Verification items for the finished model (mm, model axes). A direction names the side the tool comes from. Give positions to 0.01 mm unless a question says otherwise; leave off trailing zeros. Loops run counter-clockwise (first coordinate to the right, second up) from the corner with the lowest first, then second, coordinate; pieces in that order, holes last. Notation, with made-up numbers: (25.25, 31.5) - (61.25, 31.5) arc R33 cw to (61.25, 64.5) - close; hole circle Ø4 at (-39.75, 46). An arc over 180 degrees is marked (long way). Use one line per item in the form item = value.
```python
from build123d import *

# Parameters (mm, degrees)
PAD_DEPTH          = 10
POLARPATTERN_COUNT = 10


with BuildPart() as part:
    # Sketch002 → Pad (new body)
    with BuildSketch(Plane.XY):
        with BuildLine():
            Line((8.292424, -6.024799), (8.12043, -6.261529))
            ThreePointArc((8.12043, -6.261529), (7.99536, -6.563475), (8.021002, -6.889291))
            Line((8.021002, -6.889291), (8.744966, -9.117423))
            ThreePointArc((8.490676, -9.900046), (8.744966, -9.550046), (8.744966, -9.117423))
            Line((8.490676, -9.900046), (6.79174, -11.134395))
            ThreePointArc((5.968841, -11.134395), (6.380291, -11.268084), (6.79174, -11.134395))
            Line((5.968841, -11.134395), (4.073479, -9.757334))
            ThreePointArc((4.073479, -9.757334), (3.771533, -9.632264), (3.445717, -9.657906))
            Line((3.445717, -9.657906), (3.167424, -9.748329))
            Line((0, 0), (3.167424, -9.748329))
            Line((0, 0), (8.292424, -6.024799))
        make_face()
    pad = extrude(amount=PAD_DEPTH)

    # PolarPattern: Pad ×10 about axis
    polarpattern_axis = Axis((0, 0, 0), (0, 0, 1))
    for i in range(1, POLARPATTERN_COUNT):
        add(pad.rotate(polarpattern_axis, i * 360 / POLARPATTERN_COUNT))


solid = part.part
```
1. Tool access check on faces 1 (the flat face through (-2.08, 11.39, 4.93)), 2 (the flat face through (10, 5.5, 5)), 3 (the flat face through (2.08, -11.39, 4.93)). Record the directions out of +Z, -Z, +X, -X, +Y, -Y that give a thin tool (end or side, any length) a straight path to the whole face; none if there is none.
Result set:
face_1 = +Z, -Z, +Y
face_2 = +Z, -Z, +X, +Y
face_3 = +Z, -Z, -Y
2. Section check B-B, the plane y = 8.75. Record the cut outline in (x, z), then the cut area to 3 significant figures.
Result set:
outline = (-8.63, 0) - (8.63, 0) - (8.63, 10) - (-8.63, 10) - close
area = 173 mm²
3. Section check A-A, the plane x = 9.5. Record the cut outline in (y, z), then the cut area to 3 significant figures.
Result set:
outline = (-5.5, 0) - (5.5, 0) - (5.5, 10) - (-5.5, 10) - close
area = 110 mm²
4. Depth check by flat-ended pin: pin 1 Ø1.9 at (x, z) = (-10.5, 7) entering from +Y; pin 2 Ø4 at (x, z) = (-9, 4) entering from -Y; pin 3 Ø2 at (x, z) = (6, 5.5) entering from +Y. Enter the tip coordinate at first touch or a pass-through.
Result set:
pin_1 = 5.5
pin_2 = -10.98
pin_3 = 11.27
5. Scan lines: probe 1 along X at (y, z) = (11, 5.5); probe 2 along Y at (x, z) = (-3.75, 2.5); probe 3 along Y at (x, z) = (-9.5, 4.25). Record each from-to range of solid material in increasing order.
Result set:
probe_1 = -6.98 to -5.78, -2.21 to 2.21, 5.78 to 6.98
probe_2 = -9.63 to 9.63
probe_3 = -5.5 to 5.5
6. Draft check along Y on faces 4 (the flat face through (-10, 5.5, 5)), 5 (the flat face through (-2.07, -11.42, 4.93)), 6 (the flat face through (8.38, -7.99, 4.93)). Enter one of: released by +Y, released by -Y, zero draft, split by the parting line, or undercut.
Result set:
face_4 = released by +Y
face_5 = released by -Y
face_6 = undercut
